Can you work these out from the model? Positions are in its coordinate system, mm. Face numbers are marked on the shaded views. A direction names the side the tool comes from. Coordinates: 2 decimals unless noted, no trailing zeros. Order: outer loops, then holes, each group sorted by start corner. A loop starts at its lowest first (then second) coordinate and runs counter-clockwise, first axis right, second up. Notation, with made-up numbers: (-5.5, 17) - (50.5, 17) arc R21 cw to (50.5, 55) - close; hole circle Ø7 at (-35.5, -30). An arc over 180 degrees is marked (long way). Use a Markdown table: item, result. Add a question column.
(1) For pin 1 Ø3 at (x, y) = (1.5, -5.5) entering from +Z; pin 2 Ø7 at (x, y) = (0, 1.5) entering from +Z; pin 3 Ø4.5 at (x, z) = (-2, 12.5) entering from +Y; pin 4 Ø11 at (x, y) = (-5, 6.5) entering from +Z, each with a flat end and sliding along its axis, tell me the tip position at first contact or that it passes through.
(2) I want a section at B-B (x = 0). List the corners of the cut face in (y, z) for me, and give its area (3 significant figures).
(3) If I drill on L1, parallel to Y at x = 0, z = 4.1; L2, parallel to Y at x = 0, z = 18.25; L3, parallel to X at y = 8, z = 17, over which ranges is the centre line in solid material (lowest first)? Write a range as [from, to].
(4) We'd pull the mould along Y, two halves only. Please class the marked faces 4, 5, 6 and 7: pulls with the +Y half, pulls with the -Y half, needs draft (parallel to the pull), parting line crosses it, or undercut.
(5) On a 3-axis mill with a long thin cutter (end or side, diameter ignored), from which of +Z, -Z, +X, -X, +Y, -Y can I reach the whole of each face in a straight line? I mean the marked faces 1, 2 and 3. Say none if no direction works.
(6) I want a section at A-A (y = 1.5). List the corners of the cut face in (x, z) for me, and give its area (3 significant figures).
(7) I want a section at C-C (z = 13.25). List the corners of the cut face in (x, y) for me, and give its area (4 significant figures).
(8) I want a section at D-D (y = -13). List the corners of the cut face in (x, z) for me.
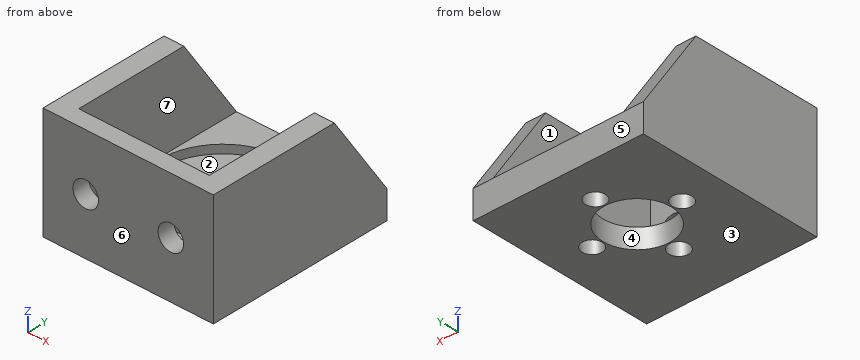
```python
from build123d import *

# Parameters (mm, degrees)
SKETCH1_W           = 30
SKETCH1_H           = 33
BOSS_EXTRUDE1_DEPTH = 5
BOSS_EXTRUDE2_DEPTH = 15
CUT_EXTRUDE1_DEPTH  = 40.651607786
SKETCH4_R           = 6
SKETCH4_R_2         = 1.75
CUT_EXTRUDE2_DEPTH  = 27.874709301
SKETCH5_R           = 11.1989
CUT_EXTRUDE3_DEPTH  = 1.5
SKETCH6_R           = 2.25
CUT_EXTRUDE4_DEPTH  = 40.05124838


with BuildPart() as part:
    # Sketch1 → Boss-Extrude1 (new body)
    with BuildSketch(Plane.XY):
        Rectangle(SKETCH1_W, SKETCH1_H)
    extrude(amount=BOSS_EXTRUDE1_DEPTH)

    # Sketch2 → Boss-Extrude2 (add)
    with BuildSketch(Plane.XY.offset(5)):
        Polygon((-15, 16.5), (-15, -16.5), (15, -16.5), (15, 16.5), (11.5, 16.5), (11.5, -13.5), (-11.5, -13.5), (-11.5, 16.5), align=None)
    extrude(amount=BOSS_EXTRUDE2_DEPTH)

    # Sketch3 → Cut-Extrude1 (cut, through all)
    with BuildSketch(Plane(origin=(15, 0, 0), x_dir=(0, 0, -1), z_dir=(1, 0, 0))):
        Polygon((-5, 16.5), (-20, 16.5), (-20, 6.5), align=None)
    extrude(amount=-CUT_EXTRUDE1_DEPTH, mode=Mode.SUBTRACT)

    # Sketch4 → Cut-Extrude2 (cut, through all)
    with BuildSketch(Plane.XY.offset(5)):
        with Locations((0, 1.5)):
            Circle(SKETCH4_R)
        with Locations((0, 9.43405)):
            Circle(SKETCH4_R_2)
        with Locations((-7.93405, 1.5)):
            Circle(SKETCH4_R_2)
        with Locations((7.93405, 1.5)):
            Circle(SKETCH4_R_2)
        with Locations((0, -6.43405)):
            Circle(SKETCH4_R_2)
    extrude(amount=-CUT_EXTRUDE2_DEPTH, mode=Mode.SUBTRACT)

    # Sketch5 → Cut-Extrude3 (cut)
    with BuildSketch(Plane.XY.offset(5)):
        with Locations((0, 1.5)):
            Circle(SKETCH5_R)
    extrude(amount=-CUT_EXTRUDE3_DEPTH, mode=Mode.SUBTRACT)

    # Sketch6 → Cut-Extrude4 (cut, through all)
    with BuildSketch(Plane(origin=(0, -13.5, 0), x_dir=(1, 0, 0), z_dir=(0, 1, 0))):
        with Locations(Location((-7.5, -10, 0), (0, 0, 180))):
            Circle(SKETCH6_R)
        with Locations(Location((7.5, -10, 0), (0, 0, 180))):
            Circle(SKETCH6_R)
    extrude(amount=-CUT_EXTRUDE4_DEPTH, mode=Mode.SUBTRACT)


solid = part.part
```
Answers follow:
| question | item | result |
|---|---|---|
| 1 | pin 1 | stops at z = 3.5 |
| 1 | pin 2 | passes through |
| 1 | pin 3 | stops at y = -13.5 |
| 1 | pin 4 | stops at z = 5 |
| 2 | outline | (-16.5, 0) - (-8.18, 0) - (-8.18, 3.5) - (-9.7, 3.5) - (-9.7, 5) - (-13.5, 5) - (-13.5, 20) - (-16.5, 20) - close; (-4.68, 0) - (-4.5, 0) - (-4.5, 3.5) - (-4.68, 3.5) - close; (7.5, 0) - (7.68, 0) - (7.68, 3.5) - (7.5, 3.5) - close; (11.18, 0) - (16.5, 0) - (16.5, 5) - (12.7, 5) - (12.7, 3.5) - (11.18, 3.5) - close |
| 2 | area | 110 mm² |
| 3 | L1 | y = [-16.5, -9.7], [12.7, 16.5] |
| 3 | L2 | y = [-16.5, -13.5] |
| 3 | L3 | x = [-15, -11.5], [11.5, 15] |
| 4 | face 4 | undercut |
| 4 | face 5 | pulls with the +Y half |
| 4 | face 6 | pulls with the -Y half |
| 4 | face 7 | needs draft |
| 5 | face 1 | +Z, +Y |
| 5 | face 2 | +Z |
| 5 | face 3 | -Z, +X, -X, +Y, -Y |
| 6 | outline | (-15, 0) - (-9.68, 0) - (-9.68, 3.5) - (-11.2, 3.5) - (-11.2, 5) - (-11.5, 5) - (-11.5, 20) - (-15, 20) - close; (-6.18, 0) - (-6, 0) - (-6, 3.5) - (-6.18, 3.5) - close; (6, 0) - (6.18, 0) - (6.18, 3.5) - (6, 3.5) - close; (9.68, 0) - (15, 0) - (15, 20) - (11.5, 20) - (11.5, 5) - (11.2, 5) - (11.2, 3.5) - (9.68, 3.5) - close |
| 6 | area | 155 mm² |
| 7 | outline | (-15, -16.5) - (15, -16.5) - (15, 11) - (11.5, 11) - (11.5, -13.5) - (-11.5, -13.5) - (-11.5, 11) - (-15, 11) - close |
| 7 | area | 261.5 mm² |
| 8 | outline | (-15, 0) - (15, 0) - (15, 20) - (11.5, 20) - (11.5, 5) - (-11.5, 5) - (-11.5, 20) - (-15, 20) - close |
